Build history of the part. All positions in model axes, mm. Face numbers are marked on the shaded views. A direction names the side the tool comes from. Give positions to 0.01 mm unless a question says otherwise; leave off trailing zeros. Write each loop counter-clockwise with the first axis right and the second up, starting at its lowest first coordinate (ties: lowest second). Pieces come first, ordered by that corner, then holes. Notation, with made-up numbers: (27, 70.5) -> (34, 70.5) arc R26 ccw to (34, 97.5) -> close; hole circle Ø1 at (58.5, -10.75). An arc over 180 degrees is marked (long way). Put each result on its own line as item: value. Start each with the question number.
Item 1: Drill centre lines: line 1 along Y through (x, z) = (-11, 2); line 2 along X through (y, z) = (-1.5, 1.55); line 3 along X through (y, z) = (-1, 2.2). Where is each one in solid material? Low to high.
Item 2: Tool access for the marked faces 1 and 2: list every direction of +Z, -Z, +X, -X, +Y, -Y with a clear straight run to the whole face (end or side of a thin tool).
Item 3: Slice it at C-C, the plane x = -5. List the corners of the cut face in (y, z).
Item 4: Flat gauge pin, fed straight in: pin 1 Ø2 at (x, z) = (-5.5, 2.5) entering from +Y. Where does the tip first touch, or does it go through?
Item 5: Slice it at D-D, the plane y = -3. List the corners of the cut face in (x, z).
Item 6: Slice it at A-A, the plane z = 3.4. Give the number of separate pieces and of enclosed holes in the cut face, plus the area to 3 significant figures.
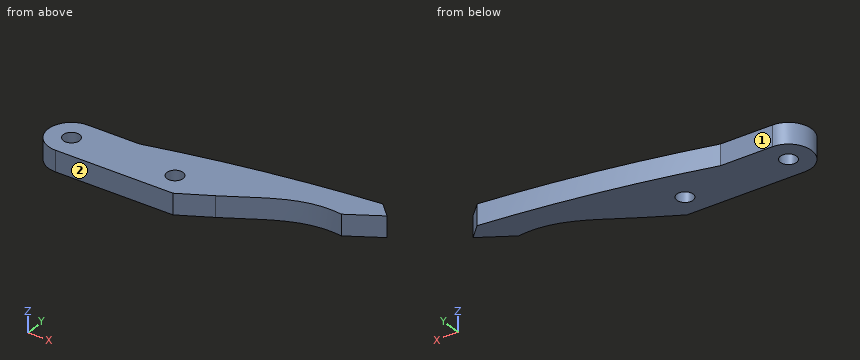
```python
from build123d import *

# Parameters (mm, degrees)
SKETCH1_R           = 5
SKETCH1_R_2         = 1.75
BOSS_EXTRUDE1_DEPTH = 4.5
BOSS_EXTRUDE2_START = -4.5
BOSS_EXTRUDE2_DEPTH = 4.5


with BuildPart() as part:
    # Sketch1 → Boss-Extrude1 (new body)
    # profile 1 of 3: a face of its own
    with BuildSketch(Plane.XY):
        with BuildLine():
            Line((-11.000000031, -5), (11, -5))
            ThreePointArc((11, -5), (6, -6e-09), (10.999999988, 5))
            Line((10.999999988, 5), (-11, 5))
            ThreePointArc((-11, 5), (-7.464466094, 3.535533906), (-6, 0))
            ThreePointArc((-6, 0), (-7.464466105, -3.535533917), (-11.000000031, -5))
        make_face()
    # profile 2 of 3: a face of its own
    with BuildSketch(Plane.XY):
        with Locations((-11, 0)):
            Circle(SKETCH1_R)
        with Locations((-11, 0)):
            Circle(SKETCH1_R_2, mode=Mode.SUBTRACT)
    # profile 3 of 3: a face of its own
    with BuildSketch(Plane.XY):
        with Locations((11, 0)):
            Circle(SKETCH1_R)
        with Locations((11, 0)):
            Circle(SKETCH1_R_2, mode=Mode.SUBTRACT)
    extrude(amount=BOSS_EXTRUDE1_DEPTH)

    # Sketch2 → Boss-Extrude2 (add)
    with BuildSketch(Plane.XY.offset(4.5).offset(BOSS_EXTRUDE2_START)):
        with BuildLine():
            Line((46.363989199, 12.87), (49.180795902, 10.03))
            Line((49.180795902, 10.03), (42.27, 6))
            add(Edge.make_bspline(
                [(42.27, 6), (33.457840426, 7.213673904), (27.801569406, 2.343916059), (20.61, -1.48)],
                knots=[0, 0, 0, 0, 1, 1, 1, 1], degree=3))
            Line((20.61, -1.48), (13.99, -5))
            Line((13.99, -5), (11, -5))
            ThreePointArc((11, -5), (16, 0), (11, 5))
            Line((11, 5), (0, 5))
            add(Edge.make_bspline(
                [(0, 5), (22.885517501, 10.707926651), (46.363989199, 12.87)],
                knots=[0, 0, 0, 1, 1, 1], degree=2))
        make_face()
    extrude(amount=BOSS_EXTRUDE2_DEPTH)


solid = part.part
```
Values follow:
1. line 1: -5 to -1.75, 1.75 to 5
1. line 2: -15.77 to -11.9, -10.1 to 10.1, 11.9 to 20.57
1. line 3: -15.9 to -12.44, -9.56 to 9.56, 12.44 to 21.5
2. face 1: +Z, -Z, -X, +Y
2. face 2: +Z, -Z, +X, -X, -Y
3. outline: (-5, 0) -> (5, 0) -> (5, 4.5) -> (-5, 4.5) -> close
4. pin 1: y = 5
5. outline: (-15, 0) -> (17.75, 0) -> (17.75, 4.5) -> (-15, 4.5) -> close
6. separate pieces: 1
6. enclosed holes: 2
6. area: 562 mm2
